Read the model definition and answer for the solid it produces. Units are mm, in the model's axes. Face numbers are marked on the shaded views. Give positions to 0.01 mm unless a question says otherwise; leave off trailing zeros. Loops run counter-clockwise (first coordinate to the right, second up) from the corner with the lowest first, then second, coordinate; pieces in that order, holes last. Notation, with made-up numbers: (82, 51) - (140, 51) arc R9 cw to (140, 62) - close; hole circle Ø6 at (-8, -22). An arc over 180 degrees is marked (long way). Write item = value, one per line.
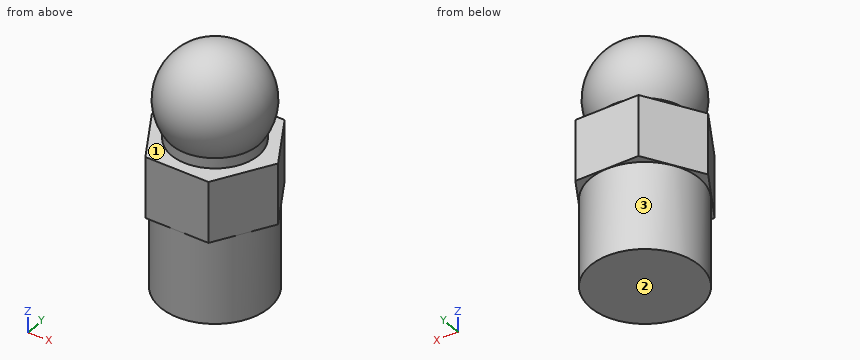
```python
from build123d import *

# Parameters (mm, degrees)
SKETCH_R     = 6.25
PAD_DEPTH    = 10
PAD001_DEPTH = 7
SKETCH002_R  = 5
PAD002_DEPTH = 8.5


with BuildPart() as part:
    # Sketch → Pad (new body)
    with BuildSketch(Plane.XY):
        Circle(SKETCH_R)
    extrude(amount=-PAD_DEPTH)

    # Sketch001 → Pad001 (join)
    with BuildSketch(Plane.XY):
        Polygon((7.274613, 0), (3.637307, 6.3), (-3.637307, 6.3), (-7.274613, 0), (-3.637307, -6.3), (3.637307, -6.3), align=None)
    extrude(amount=PAD001_DEPTH)

    # Sketch002 → Pad002 (join)
    with BuildSketch(Plane.XY):
        Circle(SKETCH002_R)
    extrude(amount=PAD002_DEPTH)

    # Sphere → Sphere (revolve)
    with BuildSketch(Plane(origin=(0, 0, 11.5), x_dir=(1, 0, 0), z_dir=(0, -1, 0))):
        with BuildLine():
            ThreePointArc((0, -6), (6, 0), (0, 6))
            Line((0, 6), (0, -6))
        make_face()
    revolve(axis=Axis((0, 0, 11.5), (0, 0, 1)))


solid = part.part
```
1) A cutting plane is placed at B-B on z = 5.5. Determine the outline of the cut face in (x, y), then the cut area to 3 significant figures.
Output:
outline = (-7.27, 0) - (-3.64, -6.3) - (3.64, -6.3) - (7.27, 0) - (3.64, 6.3) - (-3.64, 6.3) - close
area = 137 mm²
2) Each of these flat-tipped pins is pushed along its axis until it touches: P1, Ø3, axis at y = 3, z = 4, coming from the -X side; P2, Ø1, axis at y = -2.5, z = 9, coming from the -X side; P3, Ø3, axis at y = 1.5, z = 13.5, coming from the +X side; P4, Ø4, axis at x = 1, y = 1.5, coming from the +Z side. Where does it stop, or does it pass through?
Output:
P1 = -6.41
P2 = -5.18
P3 = 5.92
P4 = 17.5
3) A cutting plane is placed at A-A on x = 0. Determine the outline of the cut face in (y, z), then the cut area to 3 significant figures.
Output:
outline = (-6.3, 0) - (-6.25, 0) - (-6.25, -10) - (6.25, -10) - (6.25, 0) - (6.3, 0) - (6.3, 7) - (5, 7) - (5, 8.18) arc R6 ccw (long way) to (-5, 8.18) - (-5, 7) - (-6.3, 7) - close
area = 319 mm²
4) Find the intervals of material crossed by probe 1 along Z at (x, y) = (3.5, -5); probe 2 along X at (y, z) = (-0.25, -8.25) (3 decimals); probe 3 along Z at (x, y) = (-3.75, -5.5), in increasing order.
Output:
probe_1 = -10 to 7
probe_2 = -6.245 to 6.245
probe_3 = 0 to 7
5) A cutting plane is placed at C-C on y = -3.5. Determine the outline of the cut face in (x, z), then the cut area to 3 significant figures.
Output:
outline = (-5.25, 0) - (-5.18, 0) - (-5.18, -10) - (5.18, -10) - (5.18, 0) - (5.25, 0) - (5.25, 7) - (3.57, 7) - (3.57, 8.18) arc R4.87 ccw (long way) to (-3.57, 8.18) - (-3.57, 7) - (-5.25, 7) - close
area = 252 mm²
6) A cutting plane is placed at D-D on z = -5.5. Determine the outline of the cut face in (x, y), then the cut area to 3 significant figures.
Output:
outline = circle Ø12.5 at (0, 0)
area = 123 mm²
7) The mould has two halves that part along Z. Classify the marked faces 1, 2 and 3: pulls with the +Z half, pulls with the -Z half, needs draft (parallel to the pull), parting line crosses it, or undercut.
Output:
face_1 = undercut
face_2 = pulls with the -Z half
face_3 = needs draft
